Build history of the part. All positions in model axes, mm. Round coordinates to 2 decimals unless told otherwise and drop trailing zeros. Write each loop counter-clockwise with the first axis right and the second up, starting at its lowest first coordinate (ties: lowest second). Pieces come first, ordered by that corner, then holes. Notation, with made-up numbers: (79.5, 32) -> (93.5, 32) arc R24 cw to (93.5, 52) -> close; hole circle Ø4 at (24.5, 13). An arc over 180 degrees is marked (long way). Answer as CSV lines item,"result".
from build123d import *

# Parameters (mm, degrees)
SKETCH1_R           = 1.5
BOSS_EXTRUDE1_DEPTH = 3
SKETCH4_R           = 1.5
CUT_EXTRUDE1_DEPTH  = 5
SKETCH5_R           = 1.5
CUT_EXTRUDE2_DEPTH  = 49.645455777


with BuildPart() as part:
    # Sketch1 → Boss-Extrude1 (new body)
    with BuildSketch(Plane(origin=(0, 0, 0), x_dir=(1, 0, 0), z_dir=(0, 1, 0))):
        Polygon((35.579220967, -33.037848041), (-34.420779033, -33.037848041), (-34.420779033, 31.962151959), (-14.420779033, 31.962151959), (35.579220967, -13.037848041), align=None)
        with Locations(Location((25.579220967, -28.037848041, 0), (0, 0, 270))):
            Circle(SKETCH1_R, mode=Mode.SUBTRACT)
    extrude(amount=BOSS_EXTRUDE1_DEPTH)

    # Sketch4 → Cut-Extrude1 (cut)
    with BuildSketch(Plane(origin=(0, 3, 0), x_dir=(-1, 0, 0), z_dir=(0, 1, 0))):
        with Locations(Location((-10.579220967, 28.037848041, 0), (0, 0, 90))):
            Circle(SKETCH4_R)
    extrude(amount=-CUT_EXTRUDE1_DEPTH, mode=Mode.SUBTRACT)

    # Sketch5 → Cut-Extrude2 (cut, through all)
    with BuildSketch(Plane(origin=(0, 3, 0), x_dir=(-1, 0, 0), z_dir=(0, 1, 0))):
        with Locations(Location((24.420779033, -21.962151959, 0), (0, 0, 90))):
            Circle(SKETCH5_R)
    extrude(amount=-CUT_EXTRUDE2_DEPTH, mode=Mode.SUBTRACT)


solid = part.part
1. Cut at C-C, the plane x = -4.5. Write the cut outline in (y, z).
Results found:
outline,"(0, -23.03) -> (3, -23.03) -> (3, 33.04) -> (0, 33.04) -> close"
2. Probe line 1 along Z through (x, y) = (11.5, 0.7); line 2 along Z through (x, y) = (26, 0.45); line 3 along X through (y, z) = (2.7, -3.5). List the from-to ranges inside material, lowest first.
Results found:
line 1,"z = -8.63 to 26.85, 29.22 to 33.04"
line 2,"z = 4.42 to 26.6, 29.48 to 33.04"
line 3,"x = -34.42 to 17.2"
3. Cut at A-A, the plane z = -22. Write the cut outline in (x, y).
Results found:
outline,"(-34.42, 0) -> (-25.92, 0) -> (-25.92, 3) -> (-34.42, 3) -> close; (-22.92, 0) -> (-3.35, 0) -> (-3.35, 3) -> (-22.92, 3) -> close"
4. Mould opens along Z. For faces 1 (the cylindrical face through (24.666, 1.479, 26.847)), 2 (the flat face through (1, 1, 33.038)), 3 (the flat face through (-7, 3, 7)) say: +Z half, -Z half, draft (parallel to the pull), parting line (faces both ways), or undercut.
Results found:
face 1,"undercut"
face 2,"+Z half"
face 3,"draft"
5. Cut at D-D, the plane z = -6.5. Write the cut outline in (x, y).
Results found:
outline,"(-34.42, 0) -> (13.87, 0) -> (13.87, 3) -> (-34.42, 3) -> close"
6. Cut at B-B, the plane y = 1.1. Write the cut outline in (x, z).
Results found:
outline,"(-34.42, -31.96) -> (-14.42, -31.96) -> (35.58, 13.04) -> (35.58, 33.04) -> (-34.42, 33.04) -> close; hole circle Ø3 at (-24.42, -21.96); hole circle Ø3 at (10.58, 28.04); hole circle Ø3 at (25.58, 28.04)"
